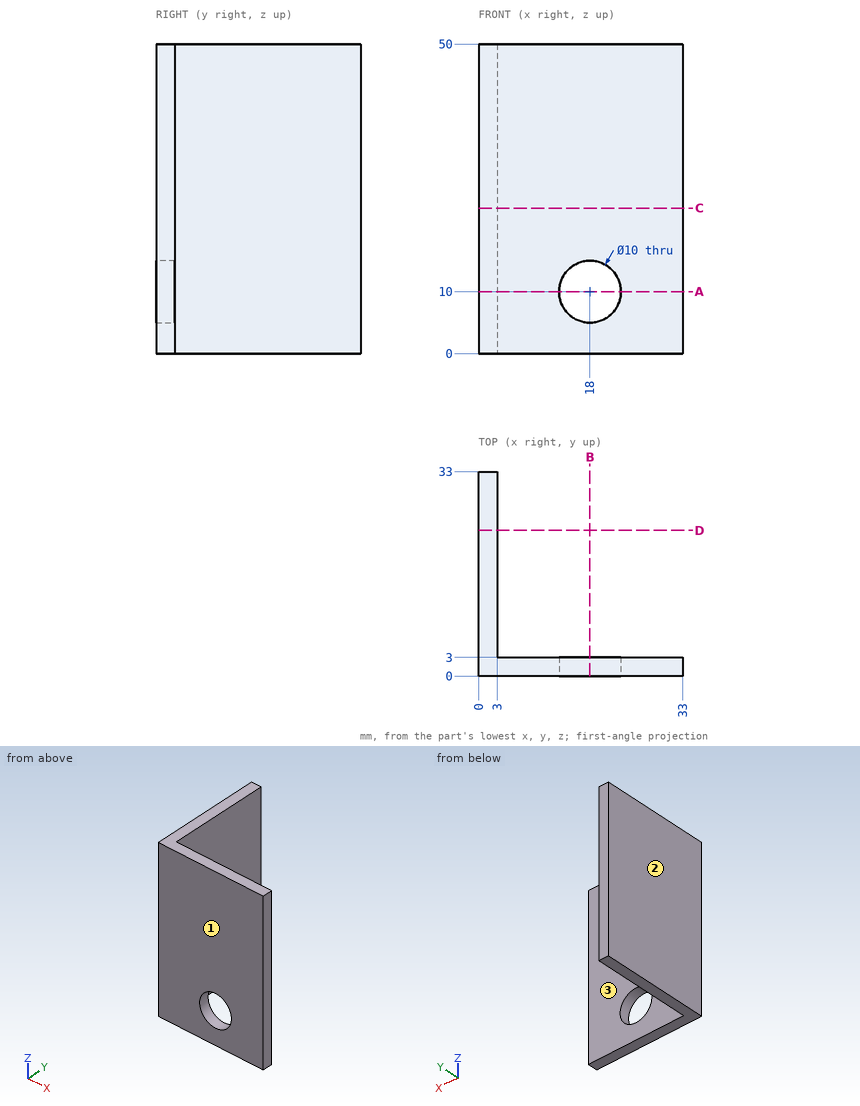
Study the drawing (mm; zero at the part's minimum x, y, z) and answer. Round coordinates to 2 decimals unless told otherwise and drop trailing zeros. Order: outer loops, then holes, each group sorted by start corner. A loop starts at its lowest first (then second) coordinate and runs counter-clockwise, first axis right, second up. Notation, with made-up numbers: M -39,58 L 15,58 A11 cw 15,63 Z; hole C 46,-4.75 d1. An arc over 180 degrees is marked long. One line per item, written item: value.
Q1. Flat-ended cylindrical pins translate along their axes: pin 1 (9 mm diameter, centred on x = 10.5, z = 30, fed in from +Y); pin 2 (13 mm diameter, centred on x = 18, z = 10, fed in from -Y); pin 3 (15 mm diameter, centred on y = 22.5, z = 37, fed in from +X). Find the tip coordinate at first contact, or state that the pin passes through.
Derived:
pin 1: y = 3
pin 2: y = 0
pin 3: x = 3
Q2. Find section C-C on z = 23.5. Write down the section's boundary in (x, y).
Derived:
outline: M 0,0 L 33,0 L 33,3 L 3,3 L 3,33 L 0,33 Z
Q3. Straight lines are drawn through the part: line 1 (X direction, y = 1, z = 10); line 2 (Z direction, x = 18, y = 1.35); line 3 (Y direction, x = 7, z = 10). For each, find the intervals that lie inside material, in ascending order.
Derived:
line 1: 0 to 13, 23 to 33
line 2: 0 to 5, 15 to 50
line 3: 0 to 3
Q4. Find section A-A on z = 10. Write down the section's boundary in (x, y).
Derived:
outline: M 0,0 L 13,0 L 13,3 L 3,3 L 3,33 L 0,33 Z; M 23,0 L 33,0 L 33,3 L 23,3 Z
Q5. Find section D-D on y = 23.5. Write down the section's boundary in (x, z).
Derived:
outline: M 0,0 L 3,0 L 3,50 L 0,50 Z
Q6. Find section B-B on x = 18. Write down the section's boundary in (y, z), then the cut area to 3 significant figures.
Derived:
outline: M 0,0 L 3,0 L 3,5 L 0,5 Z; M 0,15 L 3,15 L 3,50 L 0,50 Z
area: 120 mm²
Q7. Determine the mould class of the marked faces 1, 2 and 3 for opening direction Y: released by +Y, released by -Y, zero draft, split by the parting line, or undercut.
Derived:
face 1: released by -Y
face 2: zero draft
face 3: released by +Y
